The model under review builds one solid part; all positions refer to its coordinate system, in mm. Face numbers are marked on the shaded views. Round coordinates to 2 decimals unless told otherwise and drop trailing zeros. Loops run counter-clockwise (first coordinate to the right, second up) from the corner with the lowest first, then second, coordinate; pieces in that order, holes last. Notation, with made-up numbers: (41, 47.25) - (73, 47.25) arc R26 cw to (73, 83.25) - close; hole circle Ø8 at (72.25, 27.25). An arc over 180 degrees is marked (long way). Answer as CSV lines item,"result".
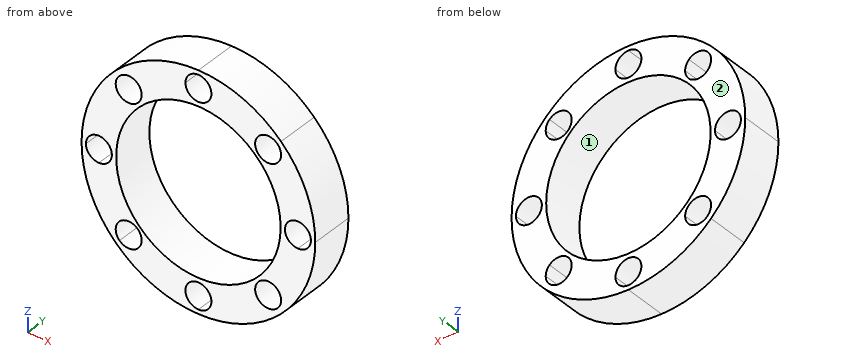
from build123d import *

# Parameters (mm, degrees)
F1_DEPTH = 1.27


with BuildPart() as f1:
    # F0 (on Front) → F1 (new body)
    with BuildSketch(Plane.XZ):
        with BuildLine():
            ThreePointArc((5.8536691527, 1.0043308473), (6.596982917, 2.1167785104), (6.858, 3.429))
            ThreePointArc((6.858, 3.429), (6.596982917, 4.7412214896), (5.8536691527, 5.8536691527))
            ThreePointArc((5.8536691527, 5.8536691527), (4.7412214896, 6.596982917), (3.429, 6.858))
            ThreePointArc((3.429, 6.858), (2.1167785104, 6.596982917), (1.0043308473, 5.8536691527))
            ThreePointArc((1.0043308473, 5.8536691527), (0.261017083, 4.7412214896), (0, 3.429))
            ThreePointArc((0, 3.429), (0.261017083, 2.1167785104), (1.0043308473, 1.0043308473))
            ThreePointArc((1.0043308473, 1.0043308473), (2.1167785104, 0.261017083), (3.429, 0))
            ThreePointArc((3.429, 0), (4.7412214896, 0.261017083), (5.8536691527, 1.0043308473))
        make_face()
        with BuildLine():
            ThreePointArc((1.7639594426, 1.3829594426), (1.5287618304, 1.0309613408), (1.113551759, 1.113551759))
            ThreePointArc((1.113551759, 1.113551759), (1.0019594426, 1.3829594426), (1.113551759, 1.6523671263))
            ThreePointArc((1.113551759, 1.6523671263), (1.5287618304, 1.7349575445), (1.7639594426, 1.3829594426))
        make_face(mode=Mode.SUBTRACT)
        with BuildLine():
            ThreePointArc((3.81, 0.508), (3.6984076836, 0.2385923164), (3.429, 0.127))
            ThreePointArc((3.429, 0.127), (3.1595923164, 0.7774076836), (3.81, 0.508))
        make_face(mode=Mode.SUBTRACT)
        with BuildLine():
            ThreePointArc((5.8560405574, 1.3829594426), (5.8270386592, 1.2371570549), (5.744448241, 1.113551759))
            ThreePointArc((5.744448241, 1.113551759), (5.0940405574, 1.3829594426), (5.744448241, 1.6523671263))
            ThreePointArc((5.744448241, 1.6523671263), (5.8270386592, 1.5287618304), (5.8560405574, 1.3829594426))
        make_face(mode=Mode.SUBTRACT)
        with BuildLine():
            ThreePointArc((0.508, 3.048), (0.2385923164, 3.1595923164), (0.127, 3.429))
            ThreePointArc((0.127, 3.429), (0.508, 3.81), (0.889, 3.429))
            ThreePointArc((0.889, 3.429), (0.7774076836, 3.1595923164), (0.508, 3.048))
        make_face(mode=Mode.SUBTRACT)
        with BuildLine():
            ThreePointArc((1.7639594426, 5.4750405574), (1.2371570549, 5.1230424555), (1.113551759, 5.744448241))
            ThreePointArc((1.113551759, 5.744448241), (1.3829594426, 5.8560405574), (1.6523671263, 5.744448241))
            ThreePointArc((1.6523671263, 5.744448241), (1.7349575445, 5.6208429451), (1.7639594426, 5.4750405574))
        make_face(mode=Mode.SUBTRACT)
        with BuildLine():
            ThreePointArc((1.016, 3.429), (3.429, 5.842), (5.842, 3.429))
            ThreePointArc((5.842, 3.429), (3.429, 1.016), (1.016, 3.429))
        make_face(mode=Mode.SUBTRACT)
        with BuildLine():
            ThreePointArc((6.35, 3.048), (6.0805923164, 3.6984076836), (6.731, 3.429))
            ThreePointArc((6.731, 3.429), (6.6194076836, 3.1595923164), (6.35, 3.048))
        make_face(mode=Mode.SUBTRACT)
        with BuildLine():
            ThreePointArc((3.048, 6.35), (3.1595923164, 6.6194076836), (3.429, 6.731))
            ThreePointArc((3.429, 6.731), (3.6984076836, 6.6194076836), (3.81, 6.35))
            ThreePointArc((3.81, 6.35), (3.429, 5.969), (3.048, 6.35))
        make_face(mode=Mode.SUBTRACT)
        with BuildLine():
            ThreePointArc((5.2056328737, 5.744448241), (5.4750405574, 5.8560405574), (5.744448241, 5.744448241))
            ThreePointArc((5.744448241, 5.744448241), (5.8270386592, 5.6208429451), (5.8560405574, 5.4750405574))
            ThreePointArc((5.8560405574, 5.4750405574), (5.3292381696, 5.1230424555), (5.2056328737, 5.744448241))
        make_face(mode=Mode.SUBTRACT)
    extrude(amount=F1_DEPTH)


solid = f1.part
1. Take a section at D-D (z = 3.25). State the section outline as (x, y) points, plus the area to 3 significant figures.
Numbers:
outline,"(0, -1.27) - (0.17, -1.27) - (0.17, 0) - (0, 0) - close; (0.84, -1.27) - (1.02, -1.27) - (1.02, 0) - (0.84, 0) - close; (5.84, -1.27) - (6.01, -1.27) - (6.01, 0) - (5.84, 0) - close; (6.69, -1.27) - (6.85, -1.27) - (6.85, 0) - (6.69, 0) - close"
area,"0.877 mm²"
2. Wall thickness on probe 1 along Z at (x, y) = (5.5, -0.15); probe 2 along Z at (x, y) = (1.25, -1); probe 3 along X at (y, z) = (-0.9, 0.5): over which ranges is each line inside the solid? List them lowest first.
Numbers:
probe 1,"z = 0.7 to 1, 1.76 to 2.19, 4.67 to 5.09, 5.86 to 6.16"
probe 2,"z = 0.78 to 1.03, 1.74 to 2.39, 4.47 to 5.12, 5.83 to 6.08"
probe 3,"x = 1.65 to 3.05, 3.81 to 5.21"
3. Take a section at A-A (x = 4.5). State the section outline as (y, z) points.
Numbers:
outline,"(-1.27, 0.17) - (0, 0.17) - (0, 1.27) - (-1.27, 1.27) - close; (-1.27, 5.59) - (0, 5.59) - (0, 6.69) - (-1.27, 6.69) - close"
4. Draft analysis for pull direction X (two halves, no side actions). For the marked faces 1 and 2, state which applies: +X half, -X half, draft (parallel to the pull), parting line (faces both ways), or undercut.
Numbers:
face 1,"undercut"
face 2,"draft"
5. Take a section at C-C (z = 2). State the section outline as (x, y) points, plus the area to 3 significant figures.
Numbers:
outline,"(0.31, -1.27) - (1.48, -1.27) - (1.48, 0) - (0.31, 0) - close; (5.37, -1.27) - (6.55, -1.27) - (6.55, 0) - (5.37, 0) - close"
area,"2.98 mm²"
6. Take a section at B-B (y = -0.9). State how many separate pieces and enclosed holes the cut face has, plus the area to 3 significant figures.
Numbers:
separate pieces,"1"
enclosed holes,"9"
area,"15.0 mm²"
